Design review of the part shown in the three views and the two pictorial views. Dimensions are in mm from the part's minimum x, y and z. Round coordinates to 2 decimals unless told otherwise and drop trailing zeros. Write each loop counter-clockwise with the first axis right and the second up, starting at its lowest first coordinate (ties: lowest second). Pieces come first, ordered by that corner, then holes. Notation, with made-up numbers: (5, -28.5) -> (30, -28.5) arc R32 cw to (30, 9.5) -> close; hole circle Ø10 at (-9, 67.5). An arc over 180 degrees is marked (long way). Answer as a JSON object with one key per item and string values. Group by question number.
1) Insertion check: pin 1 Ø23 at (x, z) = (241.3, 177.8) entering from +Y. The pin has a flat end and moves straight along its axis. Give the tip position at first contact, or say it passes through.
2) To check wall thickness, follow probe 1 along Z at (x, y) = (381, 14); probe 2 along Z at (x, y) = (132, 13.5). State the ranges of each line that lie inside material, in increasing order. Write a range as [from, to].
3) We need section D-D, the plane y = 9.75. Count the separate pieces of the cut face and the enclosed holes in it, then the cut area to 4 significant figures.
4) We need section C-C, the plane z = 88.9. Write out the cut boundary in (x, y), then the cut area to 3 significant figures.
5) We need section B-B, the plane z = 660.4. Write out the cut boundary in (x, y), then the cut area to 3 significant figures.
6) We need section A-A, the plane x = 381. Write out the cut boundary in (y, z).
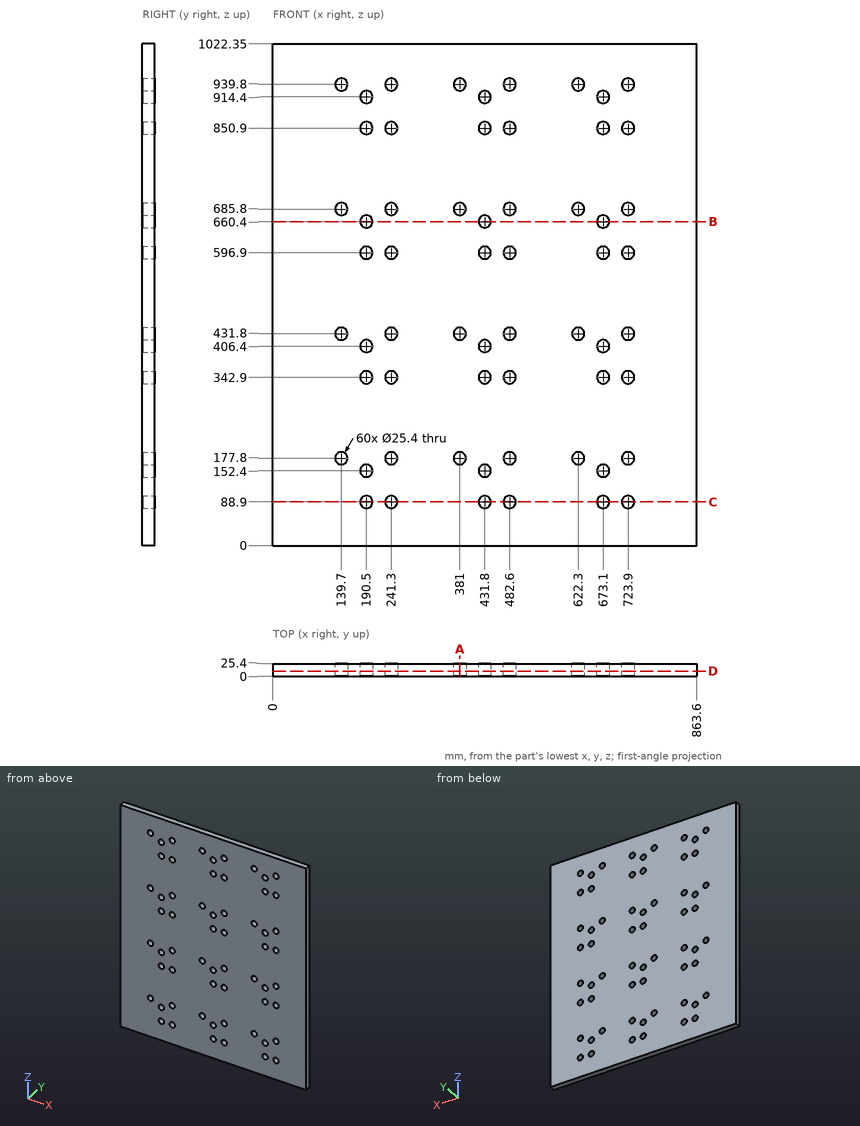
Here are the results:
{
 "1": {"pin 1": "passes through"},
 "2": {"probe 1": "z = [0, 165.1], [190.5, 419.1], [444.5, 673.1], [698.5, 927.1], [952.5, 1022.35]", "probe 2": "z = [0, 167.7], [187.9, 421.7], [441.9, 675.7], [695.9, 929.7], [949.9, 1022.35]"},
 "3": {"separate pieces": "1", "enclosed holes": "60", "area": "852,500 mm^2"},
 "4": {"outline": "(0, 0) -> (177.8, 0) -> (177.8, 25.4) -> (0, 25.4) -> close; (203.2, 0) -> (228.6, 0) -> (228.6, 25.4) -> (203.2, 25.4) -> close; (254, 0) -> (419.1, 0) -> (419.1, 25.4) -> (254, 25.4) -> close; (444.5, 0) -> (469.9, 0) -> (469.9, 25.4) -> (444.5, 25.4) -> close; (495.3, 0) -> (660.4, 0) -> (660.4, 25.4) -> (495.3, 25.4) -> close; (685.8, 0) -> (711.2, 0) -> (711.2, 25.4) -> (685.8, 25.4) -> close; (736.6, 0) -> (863.6, 0) -> (863.6, 25.4) -> (736.6, 25.4) -> close", "area": "18,100 mm^2"},
 "5": {"outline": "(0, 0) -> (177.8, 0) -> (177.8, 25.4) -> (0, 25.4) -> close; (203.2, 0) -> (419.1, 0) -> (419.1, 25.4) -> (203.2, 25.4) -> close; (444.5, 0) -> (660.4, 0) -> (660.4, 25.4) -> (444.5, 25.4) -> close; (685.8, 0) -> (863.6, 0) -> (863.6, 25.4) -> (685.8, 25.4) -> close", "area": "20,000 mm^2"},
 "6": {"outline": "(0, 0) -> (25.4, 0) -> (25.4, 165.1) -> (0, 165.1) -> close; (0, 190.5) -> (25.4, 190.5) -> (25.4, 419.1) -> (0, 419.1) -> close; (0, 444.5) -> (25.4, 444.5) -> (25.4, 673.1) -> (0, 673.1) -> close; (0, 698.5) -> (25.4, 698.5) -> (25.4, 927.1) -> (0, 927.1) -> close; (0, 952.5) -> (25.4, 952.5) -> (25.4, 1022.35) -> (0, 1022.35) -> close"}
}
